Print and shaded views of the part. All mm, measured from the part's lowest x, y and z. Round coordinates to 2 decimals unless told otherwise and drop trailing zeros. Order: outer loops, then holes, each group sorted by start corner. A loop starts at its lowest first (then second) coordinate and runs counter-clockwise, first axis right, second up.
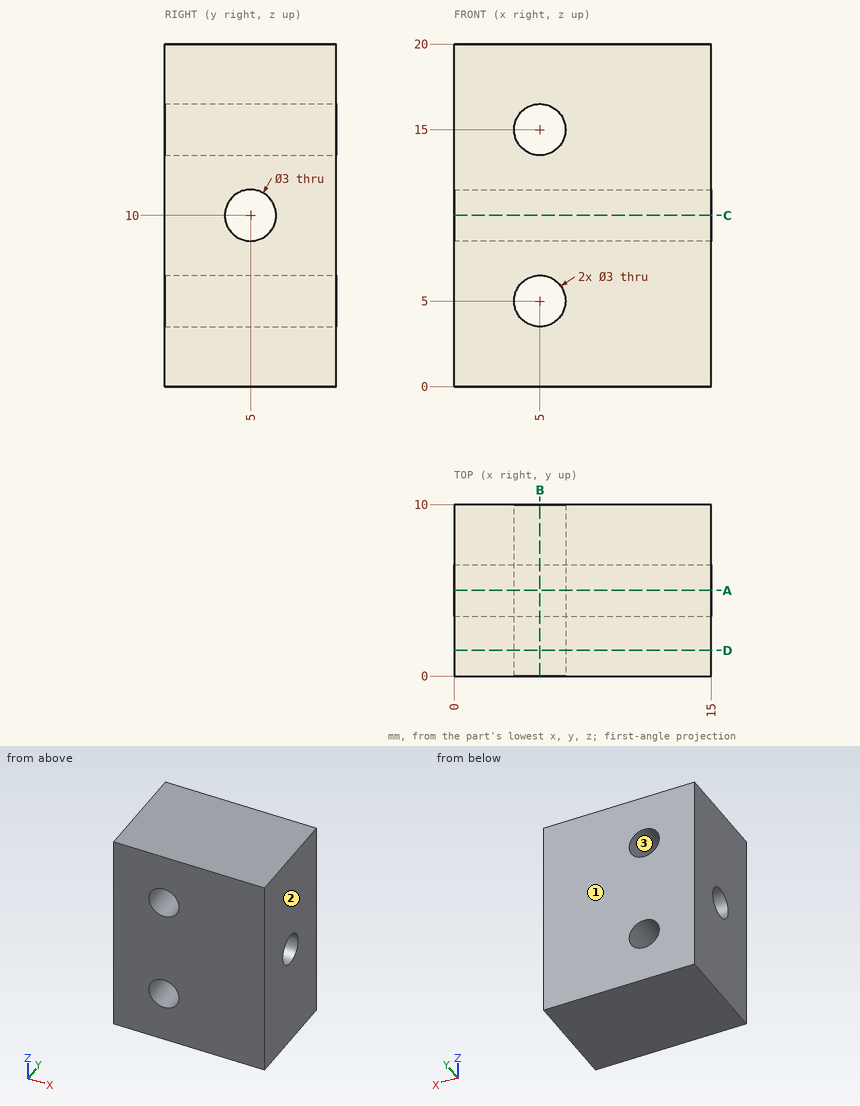
1. Cut at D-D, the plane y = 1.5. Write the cut outline in (x, z), and give its area (3 significant figures).
2. Cut at A-A, the plane y = 5. Write the cut outline in (x, z), and give its area (3 significant figures).
3. Mould opens along X. For the marked faces 1, 2 and 3 say: released by +X, released by -X, zero draft, split by the parting line, or undercut.
4. Cut at C-C, the plane z = 10. Write the cut outline in (x, y).
5. Drill centre lines: line 1 (Z direction, x = 5, y = 2.5); line 2 (X direction, y = 5.5, z = 15); line 3 (Y direction, x = 6.75, z = 10). Where is each one in solid material? Low to high.
6. Cut at B-B, the plane x = 5. Write the cut outline in (y, z), and give its area (3 significant figures).
7. Pin check, flat tips, straight feed: P1, Ø5, axis at x = 5, z = 15, coming from the -Y side; P2, Ø2.5, axis at x = 5, z = 5, coming from the +Y side. Stop position of each tip, or through.
Outcome:
1. outline: (0, 0) - (15, 0) - (15, 20) - (0, 20) - close; hole circle Ø3 at (5, 5); hole circle Ø3 at (5, 15)
1. area: 286 mm2
2. outline: (0, 0) - (15, 0) - (15, 8.5) - (0, 8.5) - close; (0, 11.5) - (15, 11.5) - (15, 20) - (0, 20) - close; hole circle Ø3 at (5, 5); hole circle Ø3 at (5, 15)
2. area: 241 mm2
3. face 1: zero draft
3. face 2: released by +X
3. face 3: undercut
4. outline: (0, 0) - (15, 0) - (15, 3.5) - (0, 3.5) - close; (0, 6.5) - (15, 6.5) - (15, 10) - (0, 10) - close
5. line 1: z = 0 to 3.5, 6.5 to 13.5, 16.5 to 20
5. line 2: x = 0 to 3.5, 6.5 to 15
5. line 3: y = 0 to 3.5, 6.5 to 10
6. outline: (0, 0) - (10, 0) - (10, 3.5) - (0, 3.5) - close; (0, 6.5) - (10, 6.5) - (10, 13.5) - (0, 13.5) - close; (0, 16.5) - (10, 16.5) - (10, 20) - (0, 20) - close; hole circle Ø3 at (5, 10)
6. area: 133 mm2
7. P1: stops at y = 0
7. P2: passes through
